from build123d import *

# Parameters (mm, degrees)
SCHIZZO1_W                   = 38
SCHIZZO1_H                   = 33.5
ESTRUSIONE_ESTRUSIONE1_DEPTH = 5
SCHIZZO2_R                   = 19
SCHIZZO2_R_2                 = 1.5
TAGLIO_ESTRUSIONE1_DEPTH     = 6


with BuildPart() as part:
    # Schizzo1 → Estrusione-Estrusione1 (new body)
    with BuildSketch(Plane(origin=(0, 0, 0), x_dir=(0, 0, -1), z_dir=(1, 0, 0))):
        Rectangle(SCHIZZO1_W, SCHIZZO1_H)
    extrude(amount=ESTRUSIONE_ESTRUSIONE1_DEPTH)

    # Schizzo2 → Taglio-Estrusione1 (cut, through all)
    with BuildSketch(Plane(origin=(0, 0, 0), x_dir=(0, 0, -1), z_dir=(1, 0, 0))):
        with Locations((0, -16.75)):
            Circle(SCHIZZO2_R)
        with Locations((-9, 11.75)):
            Circle(SCHIZZO2_R_2)
        with Locations((9, 11.75)):
            Circle(SCHIZZO2_R_2)
    extrude(amount=TAGLIO_ESTRUSIONE1_DEPTH, mode=Mode.SUBTRACT)


solid = part.part
Design review of the part built by this model. Coordinates are the model's own, in mm. Coordinates: 2 decimals unless noted, no trailing zeros. Loops run counter-clockwise (first coordinate to the right, second up) from the corner with the lowest first, then second, coordinate; pieces in that order, holes last. Notation, with made-up numbers: (-35.5, 19.5) -> (-1.5, 19.5) arc R11 cw to (-1.5, 32.5) -> close; hole circle Ø1 at (3, 11). An arc over 180 degrees is marked (long way). Use a Markdown table: item, result. Add a question column.
Item 1: We need section C-C, the plane y = 0. Write out the cut boundary in (x, z), and give its area (3 significant figures).
Item 2: We need section B-B, the plane z = 8. Write out the cut boundary in (x, y), and give its area (3 significant figures).
Item 3: We need section A-A, the plane y = 11.75. Write out the cut boundary in (x, z), and give its area (3 significant figures).
Item 4: Wall thickness on L1, parallel to Z at x = 2.8, y = 11.75; L2, parallel to Y at x = 1.9, z = 9; L3, parallel to Z at x = 3.2, y = 10.5: over which ranges is each line inside the solid? List them lowest first. Write a range as from..to.
Item 5: Clearance check with flat-ended pins moving along their axes: P1, Ø4, axis at y = 11.75, z = -9, coming from the -X side; P2, Ø3, axis at x = 2.5, z = -14.5, coming from the -Y side; P3, Ø1, axis at x = 3, z = -15, coming from the -Y side. State where each tip first meets the part, or that it passes through.
Item 6: The part is to be moulded in two halves that separate along Z. For faces 1 (the cylindrical face through (2.46, 10.84, -7.81)), 2 (the flat face through (2, 0, 19)), 3 (the flat face through (0, 8, 0)), say which applies: +Z half, -Z half, draft (parallel to the pull), parting line (faces both ways), or undercut.
Item 7: We need section D-D, the plane x = 4.45. Write out the cut boundary in (y, z).
Numbers:
| question | item | result |
|---|---|---|
| 1 | outline | (0, -19) -> (5, -19) -> (5, -8.97) -> (0, -8.97) -> close; (0, 8.97) -> (5, 8.97) -> (5, 19) -> (0, 19) -> close |
| 1 | area | 100 mm^2 |
| 2 | outline | (0, 0.48) -> (5, 0.48) -> (5, 10.63) -> (0, 10.63) -> close; (0, 12.87) -> (5, 12.87) -> (5, 16.75) -> (0, 16.75) -> close |
| 2 | area | 70.2 mm^2 |
| 3 | outline | (0, -19) -> (5, -19) -> (5, -10.5) -> (0, -10.5) -> close; (0, -7.5) -> (5, -7.5) -> (5, 7.5) -> (0, 7.5) -> close; (0, 10.5) -> (5, 10.5) -> (5, 19) -> (0, 19) -> close |
| 3 | area | 160 mm^2 |
| 4 | L1 | z = -19..-10.5, -7.5..7.5, 10.5..19 |
| 4 | L2 | y = -0.02..10.25, 13.25..16.75 |
| 4 | L3 | z = -19..-9.83, -8.17..8.17, 9.83..19 |
| 5 | P1 | stops at x = 0 |
| 5 | P2 | stops at y = -6.5 |
| 5 | P3 | stops at y = -5.76 |
| 6 | face 1 | undercut |
| 6 | face 2 | +Z half |
| 6 | face 3 | draft |
| 7 | outline | (-16.75, -19) -> (16.75, -19) -> (16.75, 19) -> (-16.75, 19) arc R19 cw to start; hole circle Ø3 at (11.75, -9); hole circle Ø3 at (11.75, 9) |
